Build history of the part. All positions in model axes, mm. Round coordinates to 2 decimals unless told otherwise and drop trailing zeros. Order: outer loops, then holes, each group sorted by start corner. A loop starts at its lowest first (then second) coordinate and runs counter-clockwise, first axis right, second up. Notation, with made-up numbers: (89, 11) - (110, 11) arc R31 cw to (110, 39) - close; hole circle Ø6 at (32, 72). An arc over 180 degrees is marked (long way). Write each question's results on one line, items separated by ' | '. Start each with the question number.
```python
from build123d import *

# Parameters (mm, degrees)
SKETCH1_R                = 35
BOSS_EXTRUDE1_DEPTH      = 5
SKETCH2_R                = 11.5
CUT_EXTRUDE1_DEPTH       = 50.749371855
SKETCH2_4_R              = 3.25
SKETCH2_4_R_2            = 1.75
CUT_EXTRUDE2_DEPTH       = 3
SKETCH2_5_R              = 1.75
CUT_EXTRUDE3_DEPTH       = 50.749371855
CIRPATTERN3_COUNT        = 4
BOSS_EXTRUDE2_START      = -5
SKETCH3_R                = 2.05
BOSS_EXTRUDE2_DEPTH      = 5
FILLET1_R                = 0.2
CIRPATTERN4_COUNT        = 4
FILLET1_OF_CIRPATTERN4_R = 0.2


with BuildPart() as part:
    # Sketch1 → Boss-Extrude1 (new body)
    with BuildSketch(Plane(origin=(0, 0, 0), x_dir=(1, 0, 0), z_dir=(0, 1, 0))):
        with Locations(Location((0, 0, 0), (0, 0, 270))):
            Circle(SKETCH1_R)
    extrude(amount=BOSS_EXTRUDE1_DEPTH)

    # Sketch2 → Cut-Extrude1 (cut, through all)
    with BuildSketch(Plane(origin=(0, 5, 0), x_dir=(1, 0, 0), z_dir=(0, 1, 0))):
        with Locations(Location((0, 0, 0), (0, 0, 270))):
            Circle(SKETCH2_R)
    extrude(amount=-CUT_EXTRUDE1_DEPTH, mode=Mode.SUBTRACT)

    # Sketch2<4> → Cut-Extrude2 (cut)
    with BuildSketch(Plane(origin=(0, 5, 0), x_dir=(1, 0, 0), z_dir=(0, 1, 0))):
        with Locations(Location((15.499780644, 15.499780644, 0), (0, 0, 270))):
            Circle(SKETCH2_4_R)
        with Locations(Location((15.499780644, 15.499780644, 0), (0, 0, 270))):
            Circle(SKETCH2_4_R_2, mode=Mode.SUBTRACT)
    cut_extrude2 = extrude(amount=-CUT_EXTRUDE2_DEPTH, mode=Mode.SUBTRACT)

    # Sketch2<5> → Cut-Extrude3 (cut, through all)
    with BuildSketch(Plane(origin=(0, 5, 0), x_dir=(1, 0, 0), z_dir=(0, 1, 0))):
        with Locations(Location((15.499780644, 15.499780644, 0), (0, 0, 270))):
            Circle(SKETCH2_5_R)
    cut_extrude3 = extrude(amount=-CUT_EXTRUDE3_DEPTH, mode=Mode.SUBTRACT)

    # CirPattern3: Cut-Extrude2, Cut-Extrude3 ×4 about axis
    cirpattern3_axis = Axis((0, 0, 0), (0, 1, 0))
    add([cut_extrude2.rotate(cirpattern3_axis, i * 360 / CIRPATTERN3_COUNT) for i in range(1, CIRPATTERN3_COUNT)], mode=Mode.SUBTRACT)
    add([cut_extrude3.rotate(cirpattern3_axis, i * 360 / CIRPATTERN3_COUNT) for i in range(1, CIRPATTERN3_COUNT)], mode=Mode.SUBTRACT)

    # Sketch3 → Boss-Extrude2 (add)
    with BuildSketch(Plane(origin=(0, 5, 0), x_dir=(1, 0, 0), z_dir=(0, 1, 0)).offset(BOSS_EXTRUDE2_START)):
        with BuildLine():
            ThreePointArc((19.664153078, 28.953774948), (24.748737342, 24.748737342), (28.953774948, 19.664153078))
            Line((28.953774948, 19.664153078), (31.335934949, 26.209083893))
            ThreePointArc((31.335934949, 26.209083893), (30.405591591, 30.405591591), (26.209083893, 31.335934949))
            Line((26.209083893, 31.335934949), (19.664153078, 28.953774948))
        make_face()
        with Locations(Location((27.577164466, 27.577164466, 0), (0, 0, 270))):
            Circle(SKETCH3_R, mode=Mode.SUBTRACT)
    boss_extrude2 = extrude(amount=BOSS_EXTRUDE2_DEPTH)

    # Fillet1
    fillet1_edges = [part.edges().sort_by_distance(p)[0] for p in [
        (19.664153078, 2.5, -28.953774948),
        (28.953774948, 2.5, -19.664153078),
    ]]
    fillet(fillet1_edges, radius=FILLET1_R)

    # CirPattern4: Boss-Extrude2 ×4 about axis
    cirpattern4_axis = Axis((0, 0, 0), (0, 1, 0))
    for i in range(1, CIRPATTERN4_COUNT):
        add(boss_extrude2.rotate(cirpattern4_axis, i * 360 / CIRPATTERN4_COUNT))

    # Fillet1 of CirPattern4
    fillet1_of_cirpattern4_edges = [part.edges().sort_by_distance(p)[0] for p in [
        (-28.953774948, 2.5, -19.664153078),
        (-19.664153078, 2.5, -28.953774948),
        (-19.664153078, 2.5, 28.953774948),
        (-28.953774948, 2.5, 19.664153078),
        (28.953774948, 2.5, 19.664153078),
        (19.664153078, 2.5, 28.953774948),
    ]]
    fillet(fillet1_of_cirpattern4_edges, radius=FILLET1_OF_CIRPATTERN4_R)


solid = part.part
```
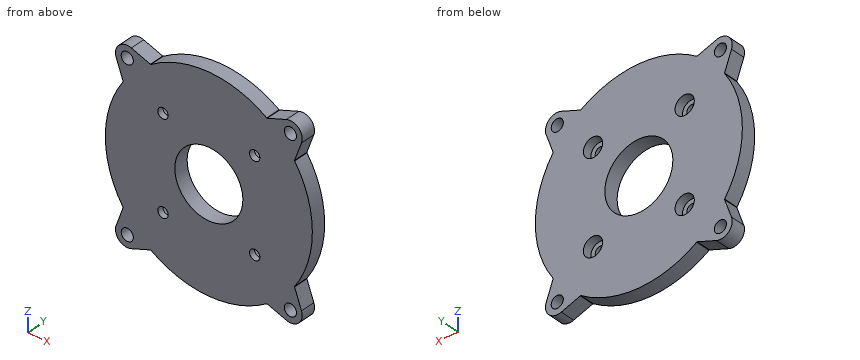
1. Cut at D-D (z = 21). List the corners of the cut face in (x, y).
2. Cut at B-B (z = 6.5). List the corners of the cut face in (x, y).
3. Cut at A-A (x = 0). List the corners of the cut face in (y, z).
4. Flat gauge pins, fed straight in: pin 1 Ø3 at (x, z) = (-15.5, 15.5) entering from -Y; pin 2 Ø1.5 at (x, y) = (24, 2) entering from -Z; pin 3 Ø3 at (x, z) = (15, -15) entering from +Y; pin 4 Ø2 at (y, z) = (1, 14) entering from +X. Where does each tip first touch, or does it go through?
5. Cut at C-C (y = 4.1). Give the number of separate pieces and of enclosed holes in the cut face, plus the area to 3 significant figures.
6. Wall check: line 1 (Z direction, x = -15.5, y = 2.9); line 2 (Z direction, x = 17, y = 4.6). Give the ranges that are in metal, low to high. Write a range as from..to.
A:
1) outline: (-29.44, 0) - (29.44, 0) - (29.44, 5) - (-29.44, 5) - close
2) outline: (-34.39, 0) - (-9.49, 0) - (-9.49, 5) - (-34.39, 5) - close; (9.49, 0) - (34.39, 0) - (34.39, 5) - (9.49, 5) - close
3) outline: (0, -35) - (5, -35) - (5, -11.5) - (0, -11.5) - close; (0, 11.5) - (5, 11.5) - (5, 35) - (0, 35) - close
4) pin 1: passes through | pin 2: stops at z = -30.8 | pin 3: stops at y = 2 | pin 4: stops at x = 32.5
5) separate pieces: 1 | enclosed holes: 9 | area: 3,530 mm^2
6) line 1: z = -31.38..-18.75, -12.25..12.25, 18.75..31.38 | line 2: z = -30.59..-18.38, -12.62..12.62, 18.38..30.59
